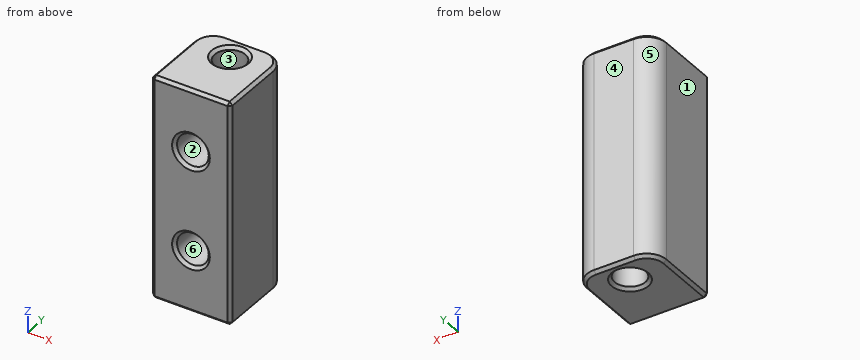
from build123d import *

# Parameters (mm, degrees)
SKETCH1_W           = 10.16
SKETCH1_H           = 28.575
SKETCH1_R           = 2.032
BOSS_EXTRUDE1_DEPTH = 10.795
SKETCH1_6_R         = 2.032
CUT_EXTRUDE3_DEPTH  = 5.08
SKETCH3_R           = 1.9685
CUT_EXTRUDE4_DEPTH  = 31.965610764
FILLET1_R           = 2.54
CHAMFER2_SIZE       = 0.381


with BuildPart() as part:
    # Sketch1 → Boss-Extrude1 (new body)
    # profile 1 of 3: a face of its own
    with BuildSketch(Plane(origin=(0, 0, 0), x_dir=(1, 0, 0), z_dir=(0, 1, 0))):
        Rectangle(SKETCH1_W, SKETCH1_H)
        with Locations((0, -6.35)):
            Circle(SKETCH1_R, mode=Mode.SUBTRACT)
        with Locations((0, 6.35)):
            Circle(SKETCH1_R, mode=Mode.SUBTRACT)
    # profile 2 of 3: a face of its own
    with BuildSketch(Plane(origin=(0, 0, 0), x_dir=(1, 0, 0), z_dir=(0, 1, 0))):
        with Locations((0, 6.35)):
            Circle(SKETCH1_R)
    # profile 3 of 3: a face of its own
    with BuildSketch(Plane(origin=(0, 0, 0), x_dir=(1, 0, 0), z_dir=(0, 1, 0))):
        with Locations((0, -6.35)):
            Circle(SKETCH1_R)
    extrude(amount=BOSS_EXTRUDE1_DEPTH)

    # Sketch1_6 → Cut-Extrude3 (cut)
    with BuildSketch(Plane(origin=(0, 0, 0), x_dir=(1, 0, 0), z_dir=(0, 1, 0))):
        with Locations(Location((0, -6.35, 0), (0, 0, 270))):
            Circle(SKETCH1_6_R)
        with Locations(Location((0, 6.35, 0), (0, 0, 270))):
            Circle(SKETCH1_6_R)
    extrude(amount=CUT_EXTRUDE3_DEPTH, mode=Mode.SUBTRACT)

    # Sketch3 → Cut-Extrude4 (cut, through all)
    with BuildSketch(Plane.XY.offset(14.2875)):
        with Locations((0, 7.62)):
            Circle(SKETCH3_R)
    extrude(amount=-CUT_EXTRUDE4_DEPTH, mode=Mode.SUBTRACT)

    # Fillet1
    fillet1_edges = [part.edges().sort_by_distance(p)[0] for p in [
        (5.08, 10.795, 0),
        (-5.08, 10.795, 0),
    ]]
    fillet(fillet1_edges, radius=FILLET1_R)

    # Chamfer2
    chamfer2_edges = [part.edges().sort_by_distance(p)[0] for p in [
        (0, 0, 4.318),
        (0, 0, -8.382),
        (-1.9685, 7.62, -14.2875),
        (-1.9685, 7.62, 14.2875),
        (0, 10.795, 14.2875),
        (0, 10.795, -14.2875),
        (-5.08, 4.1275, -14.2875),
        (5.08, 4.1275, -14.2875),
        (-4.336051224, 10.051051224, -14.2875),
        (4.336051224, 10.051051224, -14.2875),
        (5.08, 4.1275, 14.2875),
        (-5.08, 4.1275, 14.2875),
        (-4.336051224, 10.051051224, 14.2875),
        (4.336051224, 10.051051224, 14.2875),
        (0, 0, -14.2875),
        (5.08, 0, 0),
        (0, 0, 14.2875),
        (-5.08, 0, 0),
    ]]
    chamfer(chamfer2_edges, length=CHAMFER2_SIZE)


solid = part.part
Model file for the job. Use its own axes, mm. Face numbers are marked on the shaded views. A direction names the side the tool comes from. Give positions to 0.01 mm unless a question says otherwise; leave off trailing zeros. Loops run counter-clockwise (first coordinate to the right, second up) from the corner with the lowest first, then second, coordinate; pieces in that order, holes last.
1) Wall check: line 1 (X direction, y = 1.95, z = 6.35); line 2 (Y direction, x = 0, z = -7.75) (1 decimal); line 3 (Z direction, x = 1, y = 4). Give the ranges that are in metal, low to high.
2) Saw through at A-A (y = 1.25). Write the cut outline in (x, z).
3) Saw through at B-B (z = -2.25). Write the cut outline in (x, y) (1 decimal), plus the area to 3 significant figures.
4) Saw through at C-C (y = 7.62). Write the cut outline in (x, z).
5) Tool access for the marked faces 1 and 2: list every direction of +Z, -Z, +X, -X, +Y, -Y with a clear straight run to the whole face (end or side of a thin tool).
6) Saw through at D-D (x = 0). Write the cut outline in (y, z) (1 decimal), plus the area to 3 significant figures.
7) Flat gauge pins, fed straight in: pin 1 Ø1.2 at (x, z) = (-0.5, -7.5) entering from -Y; pin 2 Ø1 at (x, y) = (-1, 9) entering from +Z; pin 3 Ø2 at (y, z) = (9.5, 7.5) entering from -X. Where does each tip first touch, or does it go through?
8) Pull direction X, two halves, no side cores. Call the marked faces 3, 4, 5 and 6: +X half, -X half, draft (parallel to the pull), parting line (faces both ways), or undercut.
Answer block:
1. line 1: x = -5.08 to -2.03, 2.03 to 5.08
1. line 2: y = 5.1 to 5.7, 9.6 to 10.8
1. line 3: z = -14.29 to -8.12, -4.58 to 4.58, 8.12 to 14.29
2. outline: (-5.08, -13.91) - (-4.7, -14.29) - (4.7, -14.29) - (5.08, -13.91) - (5.08, 13.91) - (4.7, 14.29) - (-4.7, 14.29) - (-5.08, 13.91) - close; hole circle Ø4.06 at (0, -6.35); hole circle Ø4.06 at (0, 6.35)
3. outline: (-5.1, 0.4) - (-4.7, 0) - (4.7, 0) - (5.1, 0.4) - (5.1, 8.3) arc R2.5 ccw to (2.5, 10.8) - (-2.5, 10.8) arc R2.5 ccw to (-5.1, 8.3) - close; hole circle Ø3.9 at (0, 7.6)
3. area: 94.6 mm2
4. outline: (-5.08, -13.91) - (-4.7, -14.29) - (-2.35, -14.29) - (-1.97, -13.91) - (-1.97, 13.91) - (-2.35, 14.29) - (-4.7, 14.29) - (-5.08, 13.91) - close; (1.97, -13.91) - (2.35, -14.29) - (4.7, -14.29) - (5.08, -13.91) - (5.08, 13.91) - (4.7, 14.29) - (2.35, 14.29) - (1.97, 13.91) - close
5. face 1: +Z, -Z, -X, +Y, -Y
5. face 2: -Y
6. outline: (0, -13.9) - (0.4, -14.3) - (5.3, -14.3) - (5.7, -13.9) - (5.7, 13.9) - (5.3, 14.3) - (0.4, 14.3) - (0, 13.9) - (0, 8.8) - (0.4, 8.4) - (5.1, 8.4) - (5.1, 4.3) - (0.4, 4.3) - (0, 3.9) - (0, -3.9) - (0.4, -4.3) - (5.1, -4.3) - (5.1, -8.4) - (0.4, -8.4) - (0, -8.8) - close; (9.6, -13.9) - (10, -14.3) - (10.4, -14.3) - (10.8, -13.9) - (10.8, 13.9) - (10.4, 14.3) - (10, 14.3) - (9.6, 13.9) - close
6. area: 154 mm2
7. pin 1: stops at y = 5.08
7. pin 2: stops at z = 14.14
7. pin 3: stops at x = -5.07
8. face 3: undercut
8. face 4: draft
8. face 5: -X half
8. face 6: undercut
